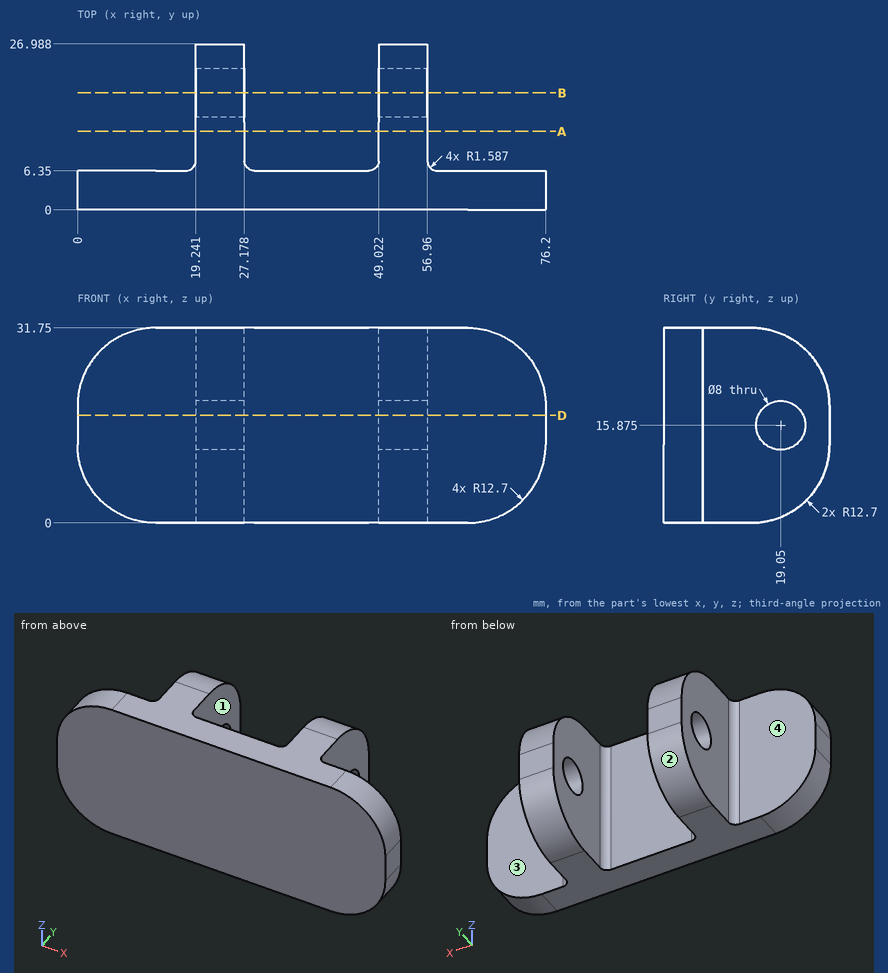
Part print with two shaded views. Sizes in mm from the minimum x, y, z corner. A direction names the side the tool comes from. Coordinates: 2 decimals unless noted, no trailing zeros. Order: outer loops, then holes, each group sorted by start corner. A loop starts at its lowest first (then second) coordinate and runs counter-clockwise, first axis right, second up. Notation, with made-up numbers: M 1,-18.75 L 8,-18.75 A28 ccw 8,14.25 Z; hole C 4.5,88.5 d4. An arc over 180 degrees is marked long. Use a Markdown table: item, result.
(1) Cut at D-D on z = 17.5. State how many separate pieces and enclosed holes the cut face has.
A:
| item | result |
|---|---|
| separate pieces | 3 |
| enclosed holes | 0 |
(2) Tool access for the marked faces 1, 2, 3 and 4: list every direction of +Z, -Z, +X, -X, +Y, -Y with a clear straight run to the whole face (end or side of a thin tool).
A:
| item | result |
|---|---|
| face 1 | +Z, -Z, +Y |
| face 2 | -Z, +X, -X, +Y |
| face 3 | +Z, -Z, +X, +Y |
| face 4 | +Z, -Z, -X, +Y |
(3) Flat gauge pins, fed straight in: pin 1 (9 mm diameter, centred on x = 6, z = 12.5, fed in from +Y); pin 2 (6 mm diameter, centred on y = 21.5, z = 7, fed in from -X); pin 3 (9.5 mm diameter, centred on x = 35, z = 15, fed in from +Y); pin 4 (7 mm diameter, centred on y = 19.05, z = 15.875, fed in from -X). Where does each tip first touch, or does it go through?
A:
| item | result |
|---|---|
| pin 1 | stops at y = 6.35 |
| pin 2 | stops at x = 19.24 |
| pin 3 | stops at y = 6.35 |
| pin 4 | passes through |
(4) Probe L1, parallel to X at y = 8, z = 27; L2, parallel to Y at x = 71, z = 5; L3, parallel to Z at x = 53, y = 16.75. List the from-to ranges inside material, lowest first.
A:
| item | result |
|---|---|
| L1 | x = 19.24 to 27.18, 49.02 to 56.96 |
| L2 | y = 0 to 6.35 |
| L3 | z = 0.24 to 12.6, 19.15 to 31.51 |
(5) Cut at A-A on y = 12.75. Write the cut outline in (x, z).
A:
| item | result |
|---|---|
| outline | M 19.24,0 L 27.18,0 L 27.18,31.75 L 19.24,31.75 Z; M 49.02,0 L 56.96,0 L 56.96,31.75 L 49.02,31.75 Z |
(6) Cut at B-B on y = 19.05. Write the cut outline in (x, z) (1 decimal).
A:
| item | result |
|---|---|
| outline | M 19.2,0.9 L 27.2,0.9 L 27.2,11.9 L 19.2,11.9 Z; M 19.2,19.9 L 27.2,19.9 L 27.2,30.8 L 19.2,30.8 Z; M 49,0.9 L 57,0.9 L 57,11.9 L 49,11.9 Z; M 49,19.9 L 57,19.9 L 57,30.8 L 49,30.8 Z |
